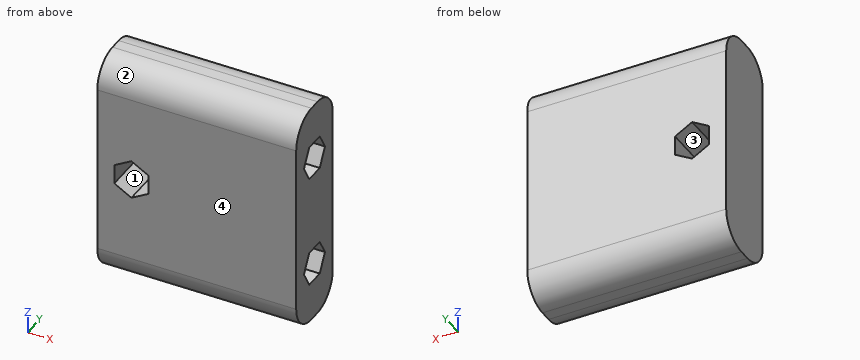
from build123d import *

# Parameters (mm, degrees)
SKETCH_2_W          = 40
SKETCH_2_H          = 12
EXTRUDE_1_DEPTH     = 35
FILLET_1_R          = 5
CUT_EXTRUDE_1_DEPTH = 20
EXTRUDE_2_DEPTH     = 10


with BuildPart() as part:
    # 草图2 → 凸台-拉伸1 (new body)
    with BuildSketch(Plane(origin=(0, 0, 0), x_dir=(0, 0, -1), z_dir=(1, 0, 0))):
        with Locations((20, 6)):
            Rectangle(SKETCH_2_W, SKETCH_2_H)
        Polygon((10, 9.464101615), (7, 7.732050808), (7, 4.267949192), (10, 2.535898385), (13, 4.267949192), (13, 7.732050808), align=None, mode=Mode.SUBTRACT)
        Polygon((30, 9.464101615), (27, 7.732050808), (27, 4.267949192), (30, 2.535898385), (33, 4.267949192), (33, 7.732050808), align=None, mode=Mode.SUBTRACT)
    extrude(amount=EXTRUDE_1_DEPTH)

    # 圆角1
    fillet_1_edges = [part.edges().sort_by_distance(p)[0] for p in [
        (17.5, 12, 0),
        (17.5, 12, -40),
        (17.5, 0, -40),
        (17.5, 0, 0),
    ]]
    fillet(fillet_1_edges, radius=FILLET_1_R)

    # 草图3 → 切除-拉伸1 (cut)
    with BuildSketch(Plane.XZ):
        Polygon((6, -16.535898385), (3, -18.267949192), (3, -21.732050808), (6, -23.464101615), (9, -21.732050808), (9, -18.267949192), align=None)
    extrude(amount=-CUT_EXTRUDE_1_DEPTH, mode=Mode.SUBTRACT)

    # 草图4 → 凸台-拉伸2 (add)
    with BuildSketch(Plane.ZY):
        Polygon((-30, 9.464101615), (-27, 7.732050808), (-27, 4.267949192), (-30, 2.535898385), (-33, 4.267949192), (-33, 7.732050808), align=None)
        Polygon((-7, 7.732050808), (-7, 4.267949192), (-10, 2.535898385), (-13, 4.267949192), (-13, 7.732050808), (-10, 9.464101615), align=None)
    extrude(amount=-EXTRUDE_2_DEPTH)


solid = part.part
Work out the finished part from the listing and answer in its coordinate system (mm). Face numbers are marked on the shaded views. Give positions to 0.01 mm unless a question says otherwise; leave off trailing zeros. Loops run counter-clockwise (first coordinate to the right, second up) from the corner with the lowest first, then second, coordinate; pieces in that order, holes last. Notation, with made-up numbers: (70.5, 14.5) - (85.5, 14.5) arc R10 cw to (85.5, 29.5) - close; hole circle Ø1 at (10, 84). An arc over 180 degrees is marked (long way). Answer in a Markdown table with one row per item. Add a question column.
Q1. The part is cut by section A-A (z = -19.5). Determine the outline of the cut face in (x, y).
Q2. The part is cut by section B-B (x = 13). Determine the outline of the cut face in (y, z), and give its area (3 significant figures).
Q3. Each of these flat-tipped pins is pushed along its axis until it touches: P1, Ø1, axis at x = 30, y = 8, coming from the +Z side; P2, Ø4, axis at y = 6.5, z = -20, coming from the -X side; P3, Ø1.8, axis at y = 7.5, z = -9.5, coming from the +X side. Where does it stop, or does it pass through?
Q4. The part is cut by section D-D (x = 9.5). Determine the outline of the cut face in (y, z), and give its area (3 significant figures).
Q5. Determine the mould class of the marked faces 1, 2, 3 and 4 for opening direction Z: released by +Z, released by -Z, zero draft, split by the parting line, or undercut.
Q6. The part is cut by section C-C (y = 5.75). Determine the outline of the cut face in (x, z), and give its area (3 significant figures).
Q7. Consider line 1 along Z through (x, y) = (27.5, 6.25); line 2 along Z through (x, y) = (16.5, 8.75); line 3 along X through (y, z) = (11, -18). Determine where each line is inside the solid, lowest interval first.
Solution:
| question | item | result |
|---|---|---|
| 1 | outline | (0, 0) - (3, 0) - (3, 12) - (0, 12) - close; (9, 0) - (35, 0) - (35, 12) - (9, 12) - close |
| 2 | outline | (0, -35) arc R5 ccw to (5, -40) - (7, -40) arc R5 ccw to (12, -35) - (12, -5) arc R5 ccw to (7, 0) - (5, 0) arc R5 ccw to (0, -5) - close; hole (2.54, -30) - (4.27, -33) - (7.73, -33) - (9.46, -30) - (7.73, -27) - (4.27, -27) - close; hole (2.54, -10) - (4.27, -13) - (7.73, -13) - (9.46, -10) - (7.73, -7) - (4.27, -7) - close |
| 2 | area | 396 mm² |
| 3 | P1 | stops at z = -0.03 |
| 3 | P2 | stops at x = 0 |
| 3 | P3 | stops at x = 10 |
| 4 | outline | (0, -35) arc R5 ccw to (5, -40) - (7, -40) arc R5 ccw to (12, -35) - (12, -5) arc R5 ccw to (7, 0) - (5, 0) arc R5 ccw to (0, -5) - close |
| 4 | area | 459 mm² |
| 5 | face 1 | undercut |
| 5 | face 2 | released by +Z |
| 5 | face 3 | undercut |
| 5 | face 4 | zero draft |
| 6 | outline | (0, -40) - (35, -40) - (35, -33) - (10, -33) - (10, -27) - (35, -27) - (35, -13) - (10, -13) - (10, -7) - (35, -7) - (35, 0) - (0, 0) - close; hole (3, -21.73) - (6, -23.46) - (9, -21.73) - (9, -18.27) - (6, -16.54) - (3, -18.27) - close |
| 6 | area | 1,070 mm² |
| 7 | line 1 | z = -40 to -33, -27 to -13, -7 to 0 |
| 7 | line 2 | z = -39.68 to -31.24, -28.76 to -11.24, -8.76 to -0.32 |
| 7 | line 3 | x = 0 to 3.46, 8.54 to 35 |
